Build history of the part. All positions in model axes, mm. A direction names the side the tool comes from. Coordinates: 2 decimals unless noted, no trailing zeros. Order: outer loops, then holes, each group sorted by start corner. A loop starts at its lowest first (then second) coordinate and runs counter-clockwise, first axis right, second up. Notation, with made-up numbers: (70.5, 1.5) - (103.5, 1.5) arc R16 ccw to (103.5, 15.5) - close; hole circle Ø8 at (-26.5, -36.75). An arc over 180 degrees is marked (long way). Return JSON: item names as keys, results as strings.
Solid Edge part; units mm, degrees
sketch "Sketch1" plane through (0, 0, 0) normal (0, 0, 1) x (1, 0, 0)
  line L0 (-15, -15) -> (15, -15)
  line L1 (15, -15) -> (15, 15)
  line L2 (15, 15) -> (-15, 15)
  line L3 (-15, 15) -> (-15, -15)
  dimension "D1" = 15
extrude "Protrusion1" add sketch "Sketch1" along normal blind 40
sketch "Sketch2" plane through (0, 0, 0) normal (0, 0, -1) x (0, 1, 0)
  line L0 (-20, -20) -> (20, -20)
  line L1 (20, -20) -> (20, 20)
  line L2 (20, 20) -> (-20, 20)
  line L3 (-20, 20) -> (-20, -20)
  dimension "D1" = 20
extrude "ExtrudedProtrusion_2" add sketch "Sketch2" along normal blind 10
sketch "Sketch3" plane through (0, 0, 40) normal (0, 0, 1) x (1, 0, 0)
  line L0 (-15, 9) -> (9, 9)
  line L1 (9, 9) -> (9, -15)
  line L2 (9, -15) -> (-15, -15)
  line L3 (-15, -15) -> (-15, 9)
  dimension "D1" = 15
extrude "ExtrudedCutout_1" cut sketch "Sketch3" against normal blind 30
chamfer "Chamfer_1" distance 5 angle 45 2 edges at (15, 0, 40) (0, 15, 40)
chamfer "Chamfer_2" distance 5 angle 45 4 edges at (15, 0, 0) (0, 15, 0) (-15, 0, 0) (0, -15, 0)
fillet "Round_1" radius 2 4 edges at (-20, 0, -10) (0, 20, -10) (0, -20, -10) (20, 0, -10)
hole "Hole_1" at (-5, -5, 10) direction (0, 0, -1) diameter 5.7 depth 40 tip angle 118 start chamfer 0.6 start chamfer angle 30 end chamfer 0.6 end chamfer angle 30
properties material "Polyethylene, low density"
1. Drop flat-ended pins along their axis: pin 1 (12 mm diameter, centred on y = -12.5, z = 16, fed in from +X); pin 2 (15 mm diameter, centred on x = 1, z = 24.5, fed in from -Y); pin 3 (8 mm diameter, centred on x = 0, z = 8.5, fed in from -Y). Give the stop position or say it passes through.
Check values:
{"pin 1": "x = 15", "pin 2": "y = 9", "pin 3": "y = -15.5"}
2. Cut at C-C on z = 11. Give the cut face in (x, y), plus the area to 3 significant figures.
Check values:
{"outline": "(-15, 9) - (9, 9) - (9, -15) - (15, -15) - (15, 15) - (-15, 15) - close", "area": "324 mm²"}
3. Probe L1, parallel to Y at x = -5, z = -0.75; L2, parallel to Y at x = -5, z = 2. List the from-to ranges inside material, lowest first.
Check values:
{"L1": "-20 to -7.85, -2.15 to 20", "L2": "-18 to -7.85, -2.15 to 18"}
4. Mould opens along Y. For faces 1 (the flat face through (0, -17, 3)), 2 (the flat face through (-3, 0, 10)), 3 (the cylindrical face through (-7.403, -6.532, -0.125)) say: pulls with the +Y half, pulls with the -Y half, needs draft (parallel to the pull), parting line crosses it, or undercut.
Check values:
{"face 1": "pulls with the -Y half", "face 2": "needs draft", "face 3": "undercut"}
5. Tool access for faces 4 (the flat face through (10, -15, 17)), 5 (the flat face through (15, 0, 20)), 6 (the flat face through (9, -3, 25)): list every direction of +Z, -Z, +X, -X, +Y, -Y with a clear straight run to the whole face (end or side of a thin tool).
Check values:
{"face 4": "+Z, +X, -X, -Y", "face 5": "+Z, +X, +Y, -Y", "face 6": "+Z, -X, -Y"}
